For this review, take the finished solid that the model builds, in its own axes (mm). Face numbers are marked on the shaded views. A direction names the side the tool comes from. Give positions to 0.01 mm unless a question says otherwise; leave off trailing zeros. Write each loop counter-clockwise with the first axis right and the second up, starting at its lowest first coordinate (ties: lowest second). Pieces come first, ordered by that corner, then holes.
1) For P1, Ø10, axis at x = -3.18, z = 61.5, coming from the -Y side; P2, Ø2, axis at y = -6, z = 52.5, coming from the -X side; P3, Ø1, axis at x = 32.5, y = -5.5, coming from the +Z side; P4, Ø2, axis at x = -3.5, y = -15, coming from the +Z side, all flat-tipped, find the tip position at first contact; note any pin that passes through.
2) We need section D-D on x = 23.5. Give the boundary of the cut face in (y, z).
3) Machinability: for the marked faces 4 and 5, which of the approach directions +Z, -Z, +X, -X, +Y, -Y give a long, thin tool a straight path to every point of the face, cutting with its end or side? Answer none if there is none.
4) We need section A-A on x = -5. Give the boundary of the cut face in (y, z).
5) We need section C-C on z = -32. Give the boundary of the cut face in (x, y).
6) We need section B-B on y = -7.75. Give the number of separate pieces and of enclosed holes in the cut face, and give its area (3 significant figures).
7) Wall thickness on line 1 along X through (y, z) = (-15.5, 74.5); line 2 along Z through (x, y) = (1, -5.5); line 3 along X through (y, z) = (-9.25, 60): over which ranges is each line inside the solid? List them lowest first.
8) Draft analysis for pull direction Z (two halves, no side actions). For the marked faces 1, 2 and 3, state which applies: pulls with the +Z half, pulls with the -Z half, needs draft (parallel to the pull), parting line crosses it, or undercut.
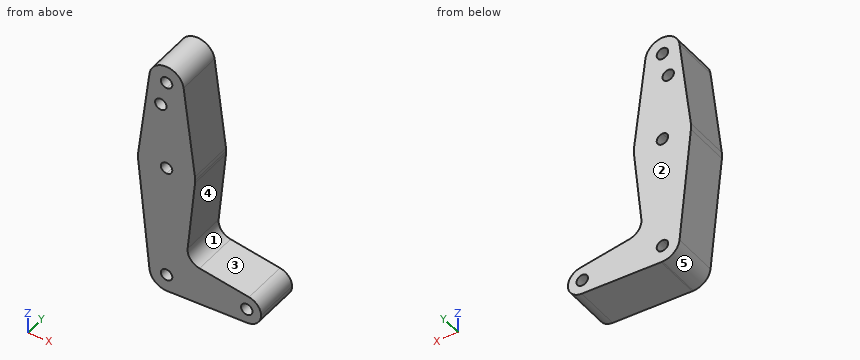
from build123d import *

# Parameters (mm, degrees)
F0_R     = 3.175
F1_DEPTH = 25.4


# Not quite as in the source:
# - a feature of the source that left no trace in its solid (it failed there, or was rolled back) is left out


with BuildPart() as f1:
    # F0 (on Front) → F1 (new body)
    with BuildSketch(Plane.XZ):
        with BuildLine():
            ThreePointArc((9.525, 75.7764706288), (6.7351920908, 69.041278538), (0, 66.2514706288))
            Line((0, 66.2514706288), (0, 61.5016706288))
            Line((0, 61.5016706288), (0, 40.8514706288))
            ThreePointArc((0, 40.8514706288), (10.5003255158, 36.8827206288), (15.7504882737, 26.9608456288))
            Line((15.7504882737, 26.9608456288), (9.4502929642, 76.9670956288))
            ThreePointArc((9.4502929642, 76.9670956288), (9.5063048942, 76.3729538708), (9.525, 75.7764706288))
        make_face()
        with BuildLine():
            ThreePointArc((-9.4502929642, 76.9670956288), (-7.14375, 69.4762753193), (0, 66.2514706288))
            ThreePointArc((0, 66.2514706288), (6.7351920908, 69.041278538), (9.525, 75.7764706288))
            ThreePointArc((9.525, 75.7764706288), (9.5063048942, 76.3729538708), (9.4502929642, 76.9670956288))
            ThreePointArc((9.4502929642, 76.9670956288), (0, 85.3014706288), (-9.4502929642, 76.9670956288))
        make_face()
        with BuildLine():
            ThreePointArc((3.175, 75.7764706288), (2.2450640303, 73.5314065985), (0, 72.6014706288))
            ThreePointArc((0, 72.6014706288), (-2.2450640303, 78.0215346591), (3.175, 75.7764706288))
        make_face(mode=Mode.SUBTRACT)
        with BuildLine():
            Line((0, 61.5016706288), (0, 66.2514706288))
            ThreePointArc((0, 66.2514706288), (-7.14375, 69.4762753193), (-9.4502929642, 76.9670956288))
            Line((-9.4502929642, 76.9670956288), (-15.7504882737, 26.9608456288))
            ThreePointArc((-15.7504882737, 26.9608456288), (-10.5003255158, 36.8827206288), (0, 40.8514706288))
            Line((0, 40.8514706288), (0, 61.5016706288))
        make_face()
        with Locations((-3.175, 61.5016706288)):
            Circle(F0_R, mode=Mode.SUBTRACT)
        with BuildLine():
            Line((0, 28.1514706288), (0, 40.8514706288))
            ThreePointArc((0, 40.8514706288), (-10.5003255158, 36.8827206288), (-15.7504882737, 26.9608456288))
            ThreePointArc((-15.7504882737, 26.9608456288), (-15.8737438155, 25.1761761155), (-15.7954255641, 23.3889706288))
            ThreePointArc((-15.7954255641, 23.3889706288), (-10.6492737428, 13.2032555305), (0, 9.1014706288))
            Line((0, 9.1014706288), (0, 21.8014706288))
            ThreePointArc((0, 21.8014706288), (-3.175, 24.9764706288), (0, 28.1514706288))
        make_face()
        with BuildLine():
            ThreePointArc((15.7504882737, 26.9608456288), (10.5003255158, 36.8827206288), (0, 40.8514706288))
            Line((0, 40.8514706288), (0, 28.1514706288))
            ThreePointArc((0, 28.1514706288), (2.2450640303, 27.2215346591), (3.175, 24.9764706288))
            ThreePointArc((3.175, 24.9764706288), (2.2450640303, 22.7314065985), (0, 21.8014706288))
            Line((0, 21.8014706288), (0, 9.1014706288))
            ThreePointArc((0, 9.1014706288), (10.6492737428, 13.2032555305), (15.7954255641, 23.3889706288))
            ThreePointArc((15.7954255641, 23.3889706288), (15.8550939106, 24.1817240747), (15.875, 24.9764706288))
            ThreePointArc((15.875, 24.9764706288), (15.8438414904, 25.9706093654), (15.7504882737, 26.9608456288))
        make_face()
        with BuildLine():
            ThreePointArc((0, 9.1014706288), (-10.6492737428, 13.2032555305), (-15.7954255641, 23.3889706288))
            Line((-15.7954255641, 23.3889706288), (-9.4772553384, -39.4760293712))
            ThreePointArc((-9.4772553384, -39.4760293712), (-7.063929059, -32.1339651255), (0, -28.9985293712))
            Line((0, -28.9985293712), (0, 9.1014706288))
        make_face()
        with BuildLine():
            ThreePointArc((15.7954255641, 23.3889706288), (10.6492737428, 13.2032555305), (0, 9.1014706288))
            Line((0, 9.1014706288), (0, -28.9985293712))
            ThreePointArc((0, -28.9985293712), (6.7351920908, -31.7883372804), (9.525, -38.5235293712))
            Line((9.525, -38.5235293712), (36.5125, -38.5235293712))
            ThreePointArc((36.5125, -38.5235293712), (39.3067692229, -32.4777801684), (45.7222218075, -30.6886485219))
            Line((45.7222218075, -30.6886485219), (18.312429941, -26.2378680158))
            ThreePointArc((18.312429941, -26.2378680158), (13.2809615783, -23.2323004998), (11.6763381809, -17.5954313572))
            Line((11.6763381809, -17.5954313572), (15.7954255641, 23.3889706288))
        make_face()
        with BuildLine():
            Line((36.5125, -38.5235293712), (9.525, -38.5235293712))
            ThreePointArc((9.525, -38.5235293712), (6.9705567315, -45.0148284595), (0.6773435479, -48.0244151572))
            Line((0.6773435479, -48.0244151572), (44.7324052746, -46.4560039858))
            ThreePointArc((44.7324052746, -46.4560039858), (38.9380895153, -44.2351621551), (36.5125, -38.5235293712))
        make_face()
        with BuildLine():
            ThreePointArc((0, -28.9985293712), (-7.063929059, -32.1339651255), (-9.4772553384, -39.4760293712))
            ThreePointArc((-9.4772553384, -39.4760293712), (-6.3895642457, -45.5874584302), (0, -48.0485293712))
            Line((0, -48.0485293712), (0.6773435479, -48.0244151572))
            ThreePointArc((0.6773435479, -48.0244151572), (6.9705567315, -45.0148284595), (9.525, -38.5235293712))
            Line((9.525, -38.5235293712), (3.175, -38.5235293712))
            ThreePointArc((3.175, -38.5235293712), (-2.2450640303, -40.7685934015), (0, -35.3485293712))
            Line((0, -35.3485293712), (0, -28.9985293712))
        make_face()
        with BuildLine():
            ThreePointArc((9.525, -38.5235293712), (6.7351920908, -31.7883372804), (0, -28.9985293712))
            Line((0, -28.9985293712), (0, -35.3485293712))
            ThreePointArc((0, -35.3485293712), (2.2450640303, -36.2784653409), (3.175, -38.5235293712))
            Line((3.175, -38.5235293712), (9.525, -38.5235293712))
        make_face()
        with BuildLine():
            ThreePointArc((45.7222218075, -30.6886485219), (39.3067692229, -32.4777801684), (36.5125, -38.5235293712))
            ThreePointArc((36.5125, -38.5235293712), (38.9380895153, -44.2351621551), (44.7324052746, -46.4560039858))
            ThreePointArc((44.7324052746, -46.4560039858), (50.1616327839, -44.0354398559), (52.3875, -38.5235293712))
            ThreePointArc((52.3875, -38.5235293712), (50.4957492028, -33.3802985941), (45.7222218075, -30.6886485219))
        make_face()
        with BuildLine():
            ThreePointArc((47.625, -38.5235293712), (44.45, -41.6985293712), (41.275, -38.5235293712))
            ThreePointArc((41.275, -38.5235293712), (44.45, -35.3485293712), (47.625, -38.5235293712))
        make_face(mode=Mode.SUBTRACT)
    extrude(amount=F1_DEPTH)


solid = f1.part
Results list:
1. P1: stops at y = -25.4
1. P2: stops at x = -12.66
1. P3: stops at z = -28.46
1. P4: stops at z = 84.97
2. outline: (-25.4, -47.21) - (0, -47.21) - (0, -27.08) - (-25.4, -27.08) - close
3. face 4: +X, +Y, -Y
3. face 5: -Z, -X, +Y, -Y
4. outline: (-25.4, -46.63) - (0, -46.63) - (0, 58.9) - (-25.4, 58.9) - close; (-25.4, 64.1) - (0, 64.1) - (0, 83.88) - (-25.4, 83.88) - close
5. outline: (-10.23, -25.4) - (48.97, -25.4) - (48.97, 0) - (-10.23, 0) - close
6. separate pieces: 1
6. enclosed holes: 5
6. area: 3,850 mm2
7. line 1: x = -9.76 to -2.91, 2.91 to 9.76
7. line 2: z = -48.01 to -41.54, -35.51 to 21.96, 27.99 to 72.76, 78.79 to 85.25
7. line 3: x = -11.59 to -5.97, -0.38 to 11.59
8. face 1: undercut
8. face 2: needs draft
8. face 3: pulls with the +Z half
